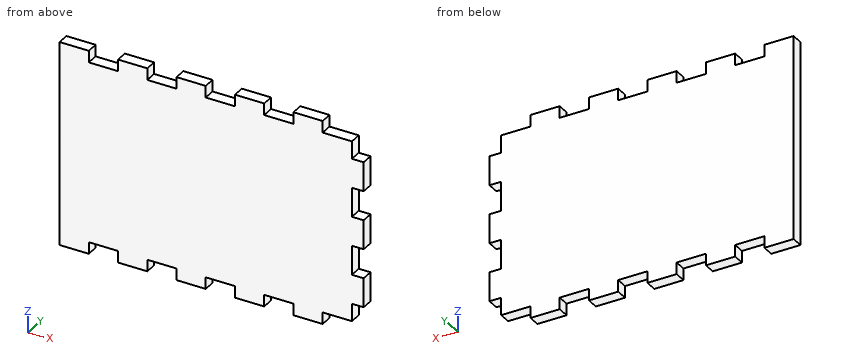
Autodesk Inventor part; units mm, degrees
ref_plane "YZ Plane" through (0, 0, 0) normal (1, 0, 0) x (0, 1, 0)
ref_plane "XZ Plane" through (0, 0, 0) normal (0, 1, 0) x (-1, 0, 0)
ref_plane "XY Plane" through (0, 0, 0) normal (0, 0, 1) x (1, 0, 0)
sketch "スケッチ1" plane through (0, 0, 0) normal (0, 1, 0) x (-1, 0, 0)
  line L0 (0, 0) -> (100, 0)
  line L1 (100, 0) -> (100, -70)
  line L2 (100, -70) -> (0, -70)
  line L3 (0, -70) -> (0, 0)
  line L4 (0, -10) -> (-4, -10)
  line L5 (-4, -10) -> (-4, -20)
  line L6 (-4, -20) -> (0, -20)
  line L7 (0, -20) -> (0, -10)
  line L8 (0, -30) -> (-4, -30)
  line L9 (-4, -30) -> (-4, -40)
  line L10 (-4, -40) -> (0, -40)
  line L11 (0, -50) -> (-4, -50)
  line L12 (-4, -50) -> (-4, -60)
  line L13 (-4, -60) -> (0, -60)
  line L14 (0, 0) -> (10, 0)
  line L15 (10, 0) -> (10, -4)
  line L16 (10, -4) -> (0, -4)
  line L17 (0, -4) -> (0, 0)
  line L18 (0, -70) -> (10, -70)
  line L19 (10, -70) -> (10, -66)
  line L20 (10, -66) -> (0, -66)
  line L21 (0, -66) -> (0, -70)
  line L22 (30, 0) -> (20, 0)
  line L23 (20, 0) -> (20, -4)
  line L24 (20, -4) -> (30, -4)
  line L25 (30, -4) -> (30, 0)
  line L26 (30, -70) -> (20, -70)
  line L27 (20, -70) -> (20, -66)
  line L28 (20, -66) -> (30, -66)
  line L29 (30, -66) -> (30, -70)
  line L30 (50, -4) -> (50, 0)
  line L31 (40, -4) -> (50, -4)
  line L32 (40, 0) -> (40, -4)
  line L33 (50, -66) -> (50, -70)
  line L34 (40, -66) -> (50, -66)
  line L35 (40, -70) -> (40, -66)
  line L36 (70, -4) -> (70, 0)
  line L37 (60, -4) -> (70, -4)
  line L38 (60, 0) -> (60, -4)
  line L39 (70, -66) -> (70, -70)
  line L40 (60, -66) -> (70, -66)
  line L41 (60, -70) -> (60, -66)
  line L42 (90, -4) -> (90, 0)
  line L43 (80, -4) -> (90, -4)
  line L44 (80, 0) -> (80, -4)
  line L45 (90, -66) -> (90, -70)
  line L46 (80, -66) -> (90, -66)
  line L47 (80, -70) -> (80, -66)
  point P0 (20, -2)
  point P1 (40, -2)
  point P2 (60, -2)
  point P3 (80, -2)
  point P4 (0, -20)
  point P5 (0, -40)
  point P6 (0, -60)
  dimension "d0" = 100
  dimension "d1" = 70
  dimension "d2" = 4
  dimension "d3" = 10
  dimension "d4" = 10
  dimension "d7" = 20
  dimension "d12" = 10
  dimension "d13" = 4
  dimension "d14" = 10
  dimension "d15" = 4
  dimension "d16" = 10
  dimension "d17" = 10
  dimension "d18" = 10
  dimension "d21" = 20
extrude "押し出し1" add sketch "スケッチ1" along normal blind 4 contours L0 L23 L24 L25 L32 L31 L30 L38 L37 L36 L44 L43 L42 L1 L2 L45 L46 L47 L39 L40 L41 L33 L34 L35 L29 L28 L27 L19 L20 L3 L16 L15 | L3 L6 L5 L4 | L3 L10 L9 L8 | L3 L13 L12 L11
properties part number "ER_lipo_back_1" material "木材 (オーク)"
Input: part model. Units: mm. Frame: model coordinates. Round coordinates to 2 decimals unless told otherwise and drop trailing zeros. Order: outer loops, then holes, each group sorted by start corner. A loop starts at its lowest first (then second) coordinate and runs counter-clockwise, first axis right, second up. Notation, with made-up numbers: (78, 21.25) - (137, 21.25) arc R33 cw to (137, 59.25) - close; hole circle Ø2 at (50, 21.5). An arc over 180 degrees is marked (long way). Answer in a Markdown table with one row per item.
Item 1: Section query B-B (z = -46.5). Return the cut outline in (x, y), then the cut area to 3 significant figures.
Model answer:
| item | result |
|---|---|
| outline | (-100, 0) - (0, 0) - (0, 4) - (-100, 4) - close |
| area | 400 mm² |
Item 2: Pin query (flat end, axial travel): pin 1 (2 mm diameter, centred on y = 3, z = -2.5, fed in from +X); pin 2 (1 mm diameter, centred on x = -87.5, y = 3, fed in from +Z); pin 3 (1.2 mm diameter, centred on x = 2, y = 2, fed in from +Z). Return the tip coordinate at first contact, or that it passes through.
Model answer:
| item | result |
|---|---|
| pin 1 | stops at x = -10 |
| pin 2 | stops at z = -4 |
| pin 3 | stops at z = -10 |
Item 3: Line query: line 1 (X direction, y = 0.4, z = -3); line 2 (Z direction, x = -85, y = 1.15); line 3 (X direction, y = 0.7, z = -6.5). Output: solid intervals per line, ascending.
Model answer:
| item | result |
|---|---|
| line 1 | x = -100 to -90, -80 to -70, -60 to -50, -40 to -30, -20 to -10 |
| line 2 | z = -66 to -4 |
| line 3 | x = -100 to 0 |
Item 4: Section query A-A (x = -88.5). Return the cut outline in (y, z), then the cut area to 3 significant figures.
Model answer:
| item | result |
|---|---|
| outline | (0, -66) - (4, -66) - (4, -4) - (0, -4) - close |
| area | 248 mm² |
